For this review, take the finished solid that the model builds, in its own axes (mm). Face numbers are marked on the shaded views. Coordinates: 2 decimals unless noted, no trailing zeros. Order: outer loops, then holes, each group sorted by start corner. A loop starts at its lowest first (then second) coordinate and runs counter-clockwise, first axis right, second up. Notation, with made-up numbers: (2, 70.5) - (38, 70.5) arc R10 ccw to (38, 87.5) - close; hole circle Ø11 at (55.5, 76). An arc over 180 degrees is marked (long way). One line per item, written item: value. Start each with the question number.
(1) Consider section D-D on x = 11.5. Write out the cut boundary in (y, z).
(2) Consider section C-C on y = 0. Write out the cut boundary in (x, z).
(3) To check wall thickness, follow line 1 along Y through (x, z) = (0, 3.3); line 2 along Y through (x, z) = (0, 0.7); line 3 along X through (y, z) = (0, 1.9). State the ranges of each line that lie inside material, in increasing order.
(4) Consider section B-B on z = 3.4. Write out the cut boundary in (x, y), then the cut area to 3 significant figures.
(5) Consider section A-A on x = 0. Write out the cut boundary in (y, z), then the cut area to 3 significant figures.
(6) Mouldability with a two-part tool opening along X and no side actions: class the marked faces 1, 2, 3 and 4 as released by +X, released by -X, zero draft, split by the parting line, or undercut.
(7) Clearance check with flat-ended pins moving along their axes: pin 1 (5 mm diameter, centred on x = 0, y = 0, fed in from +Z); pin 2 (4 mm diameter, centred on x = 16.5, y = 8.5, fed in from -Z); pin 3 (2.5 mm diameter, centred on x = 0, y = 0, fed in from +Z); pin 4 (2 mm diameter, centred on x = -12.5, z = 2, fed in from -Y). State where each tip first meets the part, or that it passes through.
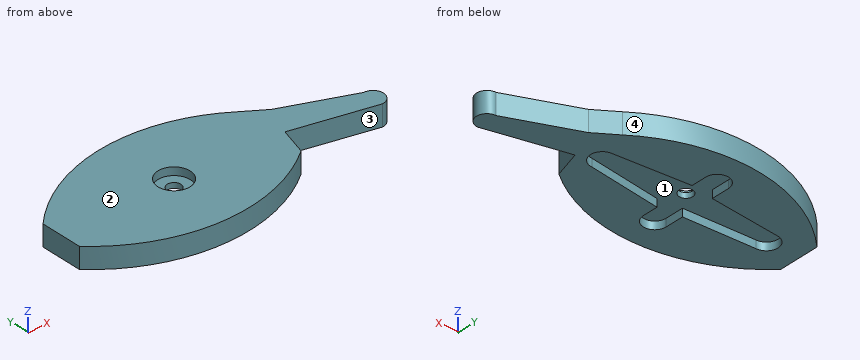
```python
from build123d import *

# Parameters (mm, degrees)
PAD_DEPTH       = 4
POCKET_DEPTH    = 1.5
SKETCH002_R     = 3.1
POCKET001_DEPTH = 1.5
SKETCH003_R     = 1.3
POCKET002_DEPTH = 4.001


with BuildPart() as part:
    # Sketch001 → Pad (new body)
    with BuildSketch(Plane.XY):
        with BuildLine():
            Line((-21.78, 0), (-21.78, 3.903012))
            ThreePointArc((18.4, 6.81485), (-2.23065, 12.819278), (-21.78, 3.903012))
            Line((18.4, 6.81485), (22.430655, 4.019184))
            Line((35.211283, -1.556892), (22.430655, 4.019184))
            ThreePointArc((35.211283, -5.556892), (37.211283, -3.556892), (35.211283, -1.556892))
            Line((35.211283, -5.556892), (19.965446, -1.596008))
            Line((18.4, -6.81485), (19.965446, -1.596008))
            ThreePointArc((-21.78, -3.903012), (-2.23065, -12.819278), (18.4, -6.81485))
            Line((-21.78, 0), (-21.78, -3.903012))
        make_face()
    extrude(amount=PAD_DEPTH)

    # Sketch → Pocket (cut)
    with BuildSketch(Plane.XY):
        with BuildLine():
            ThreePointArc((2.2, 6.7), (0, 8.9), (-2.2, 6.7))
            Line((-2.2, 3.2), (-2.2, 6.7))
            Line((-15.52, 2.26), (-2.2, 3.2))
            ThreePointArc((-15.52, 2.26), (-17.78, 0), (-15.52, -2.26))
            Line((-2.2, -3.2), (-15.52, -2.26))
            Line((-2.2, -6.7), (-2.2, -3.2))
            ThreePointArc((-2.2, -6.7), (0, -8.9), (2.2, -6.7))
            Line((2.2, -3.77), (2.2, -6.7))
            Line((16.13, -2.27), (2.2, -3.77))
            ThreePointArc((16.13, -2.27), (18.4, 0), (16.13, 2.27))
            Line((2.2, 3.77), (16.13, 2.27))
            Line((2.2, 6.7), (2.2, 3.77))
        make_face()
    extrude(amount=POCKET_DEPTH, mode=Mode.SUBTRACT)

    # Sketch002 → Pocket001 (cut)
    with BuildSketch(Plane.XY.offset(4)):
        Circle(SKETCH002_R)
    extrude(amount=-POCKET001_DEPTH, mode=Mode.SUBTRACT)

    # Sketch003 → Pocket002 (cut, through all)
    with BuildSketch(Plane.XY):
        Circle(SKETCH003_R)
    extrude(amount=POCKET002_DEPTH, mode=Mode.SUBTRACT)


solid = part.part
```
Geometry check:
1. outline: (-10.68, 0) - (-2.77, 0) - (-2.77, 1.5) - (2.77, 1.5) - (2.77, 0) - (10.68, 0) - (10.68, 4) - (-10.68, 4) - close
2. outline: (-21.78, 0) - (-17.78, 0) - (-17.78, 1.5) - (-1.3, 1.5) - (-1.3, 2.5) - (-3.1, 2.5) - (-3.1, 4) - (-21.78, 4) - close; (1.3, 1.5) - (18.4, 1.5) - (18.4, 0) - (31.64, 0) - (31.64, 4) - (3.1, 4) - (3.1, 2.5) - (1.3, 2.5) - close
3. line 1: y = -12.9 to -3.1, 3.1 to 12.9
3. line 2: y = -12.9 to -8.9, 8.9 to 12.9
3. line 3: x = -21.78 to -1.3, 1.3 to 31.64
4. outline: (-21.78, -3.9) arc R30.86 ccw to (18.4, -6.81) - (19.97, -1.6) - (35.21, -5.56) arc R2 ccw to (35.21, -1.56) - (22.43, 4.02) - (18.4, 6.81) arc R30.86 ccw to (-21.78, 3.9) - close; hole circle Ø6.2 at (0, 0)
4. area: 918 mm^2
5. outline: (-12.9, 0) - (-8.9, 0) - (-8.9, 1.5) - (-1.3, 1.5) - (-1.3, 2.5) - (-3.1, 2.5) - (-3.1, 4) - (-12.9, 4) - close; (1.3, 1.5) - (8.9, 1.5) - (8.9, 0) - (12.9, 0) - (12.9, 4) - (3.1, 4) - (3.1, 2.5) - (1.3, 2.5) - close
5. area: 64.6 mm^2
6. face 1: undercut
6. face 2: zero draft
6. face 3: undercut
6. face 4: split by the parting line
7. pin 1: stops at z = 2.5
7. pin 2: stops at z = 0
7. pin 3: passes through
7. pin 4: stops at y = -10.68
